Check sheet for the modelled part. Datum: model origin and axes. Units: mm. Coordinates: 2 decimals unless noted, no trailing zeros. Write each loop counter-clockwise with the first axis right and the second up, starting at its lowest first coordinate (ties: lowest second). Pieces come first, ordered by that corner, then holes. Notation, with made-up numbers: (49, 84.5) -> (78, 84.5) arc R18 cw to (78, 118.5) -> close; hole circle Ø10 at (-2.75, 12.25). An arc over 180 degrees is marked (long way). One line per item, written item: value. Start each with the question number.
1) Sectioned sample at D-D on z = -1. Enter the section's corners in (x, y), plus the area to 3 significant figures.
2) Scan lines: line 1 along Z through (x, y) = (12, -1.05); line 2 along X through (y, z) = (-0.4, 1.75); line 3 along X through (y, z) = (-2.35, 2). Record each from-to range of solid material in increasing order. Write a range as [from, to].
3) Sectioned sample at A-A on x = 14. Enter the section's corners in (y, z), plus the area to 3 significant figures.
4) Sectioned sample at C-C on y = -4.2. Enter the section's corners in (x, z).
5) Sectioned sample at B-B on z = -2. Enter the section's corners in (x, y), plus the area to 3 significant figures.
6) Gauge pin test, flat end, axial feed: P1, Ø3, axis at y = -3, z = 3.5, coming from the -X side. Record the tip position at first contact, or that the pin passes through.
```python
from build123d import *

# Parameters (mm, degrees)
F0_R     = 2.5
F1_DEPTH = 5


with BuildPart() as f1:
    # F0 (on Front) → F1 (new body)
    with BuildSketch(Plane.XZ):
        with BuildLine():
            ThreePointArc((0, -4.25), (3.005204, -3.005204), (4.25, 0))
            ThreePointArc((4.25, 0), (3.005204, 3.005204), (0, 4.25))
            ThreePointArc((0, 4.25), (-4.25, 0), (0, -4.25))
        make_face()
        Circle(F0_R, mode=Mode.SUBTRACT)
        with BuildLine():
            ThreePointArc((16.25, 0), (15.005204, 3.005204), (12, 4.25))
            ThreePointArc((12, 4.25), (7.75, 0), (12, -4.25))
            ThreePointArc((12, -4.25), (15.005204, -3.005204), (16.25, 0))
        make_face()
        with Locations((12, 0)):
            Circle(F0_R, mode=Mode.SUBTRACT)
        with BuildLine():
            ThreePointArc((0, 4.25), (3.005204, 3.005204), (4.25, 0))
            ThreePointArc((4.25, 0), (3.005204, -3.005204), (0, -4.25))
            Line((0, -4.25), (12, -4.25))
            ThreePointArc((12, -4.25), (7.75, 0), (12, 4.25))
            Line((12, 4.25), (0, 4.25))
        make_face()
    extrude(amount=F1_DEPTH)


solid = f1.part
```
Answers:
1. outline: (-4.13, -5) -> (-2.29, -5) -> (-2.29, 0) -> (-4.13, 0) -> close; (2.29, -5) -> (9.71, -5) -> (9.71, 0) -> (2.29, 0) -> close; (14.29, -5) -> (16.13, -5) -> (16.13, 0) -> (14.29, 0) -> close
1. area: 55.5 mm2
2. line 1: z = [-4.25, -2.5], [2.5, 4.25]
2. line 2: x = [-3.87, -1.79], [1.79, 10.21], [13.79, 15.87]
2. line 3: x = [-3.75, -1.5], [1.5, 10.5], [13.5, 15.75]
3. outline: (-5, -3.75) -> (0, -3.75) -> (0, -1.5) -> (-5, -1.5) -> close; (-5, 1.5) -> (0, 1.5) -> (0, 3.75) -> (-5, 3.75) -> close
3. area: 22.5 mm2
4. outline: (0, -4.25) -> (12, -4.25) arc R4.25 ccw to (16.25, 0) arc R4.25 ccw to (12, 4.25) -> (0, 4.25) arc R4.25 ccw to start; hole circle Ø5 at (0, 0); hole circle Ø5 at (12, 0)
5. outline: (-3.75, -5) -> (-1.5, -5) -> (-1.5, 0) -> (-3.75, 0) -> close; (1.5, -5) -> (10.5, -5) -> (10.5, 0) -> (1.5, 0) -> close; (13.5, -5) -> (15.75, -5) -> (15.75, 0) -> (13.5, 0) -> close
5. area: 67.5 mm2
6. P1: stops at x = -3.75
